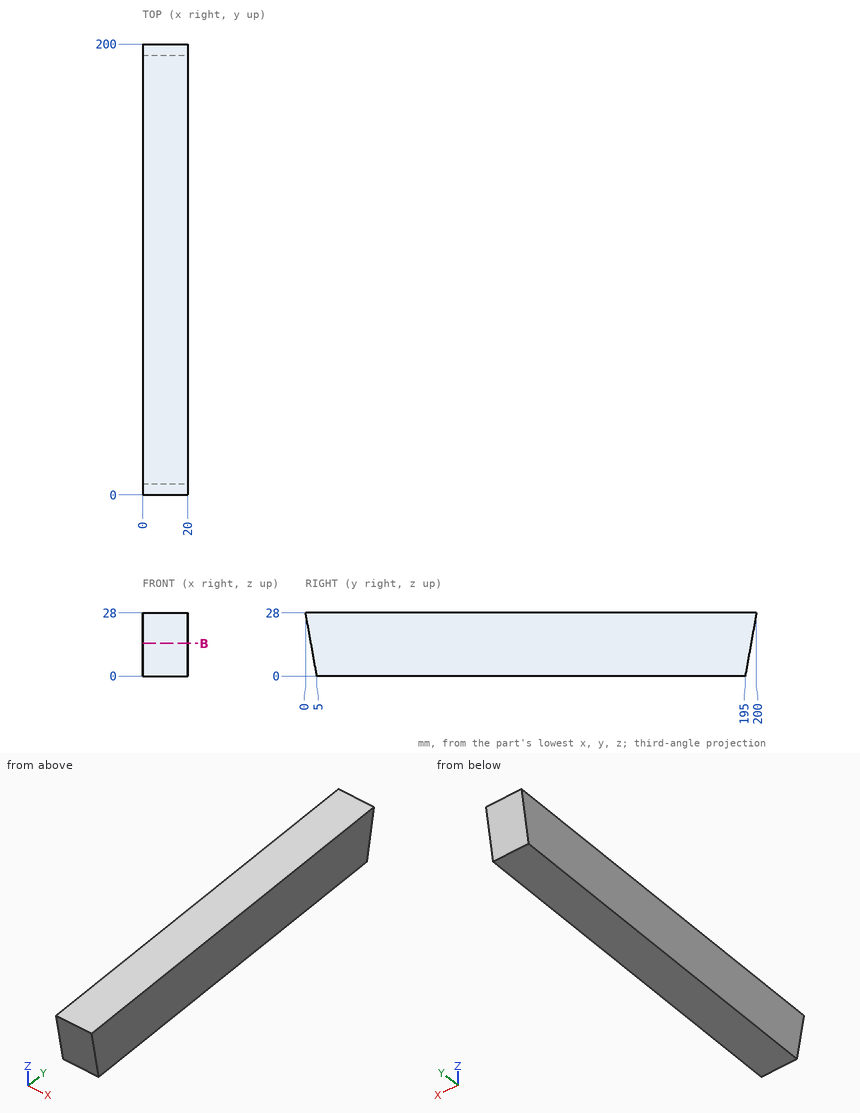
Input: dimensioned drawing with shaded views. Units: mm. Origin: part minimum x, y, z. Round coordinates to 2 decimals unless told otherwise and drop trailing zeros. Order: outer loops, then holes, each group sorted by start corner. A loop starts at its lowest first (then second) coordinate and runs counter-clockwise, first axis right, second up. Notation, with made-up numbers: (42.5, 72.25) - (78.5, 72.25) arc R17 cw to (78.5, 97.25) - close; hole circle Ø1 at (24, 43). An arc over 180 degrees is marked (long way). Answer as a JSON object with one key per item and string values. Group by question number.
(1) Pin query (flat end, axial travel): P1, Ø8, axis at x = 11, z = 9.5, coming from the -Y side; P2, Ø6, axis at y = 22, z = 15, coming from the -X side; P3, Ø10, axis at x = 16.5, z = 21, coming from the +Y side. Return the tip coordinate at first contact, or that it passes through.
(2) Cut plane B-B (z = 14.5). Return loops of the section in (x, y), then the cut area to 3 significant figures.
(3) Material intervals for probe 1 along Y at (x, z) = (4, 13); probe 2 along Y at (x, z) = (17.75, 19), sorted ascending. Write a range as from..to.
Here are the results:
{
 "1": {"P1": "stops at y = 2.59", "P2": "stops at x = 0", "P3": "stops at y = 199.64"},
 "2": {"outline": "(0, 2.41) - (20, 2.41) - (20, 197.59) - (0, 197.59) - close", "area": "3,900 mm^2"},
 "3": {"probe 1": "y = 2.68..197.32", "probe 2": "y = 1.61..198.39"}
}
